Geometry: final body of the model. Coordinates: model frame, mm. A direction names the side the tool comes from. Round coordinates to 2 decimals unless told otherwise and drop trailing zeros. Write each loop counter-clockwise with the first axis right and the second up, starting at its lowest first coordinate (ties: lowest second). Pieces come first, ordered by that corner, then holes. Notation, with made-up numbers: M -33.75,34 L -22.75,34 A19 cw -22.75,47 Z; hole C 61,72 d10. An arc over 180 degrees is marked long. Put each result on its own line as item: value. Start each with the question number.
```python
from build123d import *

# Parameters (mm, degrees)
SKETCH041_W            = 50
SKETCH041_H            = 4.45
PAD014_DEPTH           = 80
PAD013_DEPTH           = 8
SKETCH042_R            = 3
POCKET011_DEPTH        = 5
PAD011_DEPTH           = 6.5
CHAMFER_SIZE           = 2
SKETCH020_W            = 32
SKETCH020_H            = 40
POCKET004_DEPTH        = 4.5
SKETCH021_W            = 16
SKETCH021_H            = 13
POCKET005_DEPTH        = 3
POCKET006_DEPTH        = 2
PAD012_DEPTH           = 2.5
POCKET007_DEPTH        = 5
POCKET008_DEPTH        = 6.501
LINEARPATTERN001_COUNT = 6
LINEARPATTERN001_PITCH = 2.8
POCKET009_DEPTH        = 6.501
POCKET009_DEPTH_BACK   = 6.501
LINEARPATTERN002_COUNT = 6
LINEARPATTERN002_PITCH = 3.2


with BuildPart() as separation_top:
    # Sketch041 → Pad014 (new body)
    with BuildSketch(Plane.XZ.offset(2)):
        with Locations((0, 4.775)):
            Rectangle(SKETCH041_W, SKETCH041_H)
    extrude(amount=-PAD014_DEPTH)

    # AdditivePipe: sweep along a path in Sketch033
    with BuildLine(Plane.XY) as additivepipe_path:
        Line((5.5, 0.7), (15.664513, 0.7))
        ThreePointArc((15.664513, 0.7), (16.796157, 1.050945), (17.530656, 1.980617))
        ThreePointArc((17.530656, 1.980617), (20.610558, 39.551278), (2.853097, 72.80354))
        ThreePointArc((2.853097, 72.80354), (1e-05, 74), (-2.853084, 72.803553))
        ThreePointArc((-2.853084, 72.803553), (-20.610556, 39.551287), (-17.530656, 1.980617))
        ThreePointArc((-17.530656, 1.980617), (-16.796157, 1.050945), (-15.664513, 0.7))
        Line((-15.664513, 0.7), (-5.5, 0.7))
    # Sketch032 → AdditivePipe (sweep)
    with BuildSketch(Plane.YZ):
        Polygon((75.182615, 3), (72.817385, 3), (73.75, 1), (74.25, 1), align=None)
    sweep(path=additivepipe_path.line)

    # Sketch040 → Pad013 (join)
    with BuildSketch(Plane.XY.offset(-2)):
        with BuildLine():
            ThreePointArc((-4.584919, 45.32271), (-5.584919, 44.32271), (-4.584919, 43.32271))
            Line((-4.584919, 43.32271), (4.584919, 43.32271))
            ThreePointArc((4.584919, 43.32271), (5.584919, 44.32271), (4.584919, 45.32271))
            Line((4.584919, 45.32271), (-4.584919, 45.32271))
        make_face()
    extrude(amount=PAD013_DEPTH)

    # Sketch042 → Pocket011 (cut)
    with BuildSketch(Plane.XY):
        with Locations((19, 20)):
            Circle(SKETCH042_R)
        with Locations((-19, 20)):
            Circle(SKETCH042_R)
        with Locations((0, 70)):
            Circle(SKETCH042_R)
    extrude(amount=POCKET011_DEPTH, mode=Mode.SUBTRACT)


with BuildPart() as top_housing:
    # Sketch019 → Pad011 (new body, symmetric)
    with BuildSketch(Plane.XY):
        with BuildLine():
            ThreePointArc((4.279646, 74.20531), (0, 76), (-4.279646, 74.20531))
            ThreePointArc((-4.279646, 74.20531), (-22.568944, 39.95714), (-19.396798, 1.261235))
            ThreePointArc((-19.396798, 1.261235), (-17.9278, -0.59811), (-15.664513, -1.3))
            Line((15.664513, -1.3), (-15.664513, -1.3))
            ThreePointArc((15.664513, -1.3), (17.927792, -0.598116), (19.396791, 1.261217))
            ThreePointArc((19.396791, 1.261217), (22.568946, 39.95713), (4.279646, 74.20531))
        make_face()
    extrude(amount=PAD011_DEPTH, both=True)

    # Chamfer
    chamfer_edges = [top_housing.edges().sort_by_distance(p)[0] for p in [
        (0, -1.3, 6.5),
        (0, -1.3, -6.5),
    ]]
    chamfer(chamfer_edges, length=CHAMFER_SIZE)

    # Sketch020 → Pocket004 (cut)
    with BuildSketch(Plane.XY):
        with Locations((0, 20)):
            Rectangle(SKETCH020_W, SKETCH020_H)
    extrude(amount=POCKET004_DEPTH, mode=Mode.SUBTRACT)

    # Sketch021 → Pocket005 (cut)
    with BuildSketch(Plane.XY):
        with Locations((0, 57)):
            Rectangle(SKETCH021_W, SKETCH021_H)
    extrude(amount=POCKET005_DEPTH, mode=Mode.SUBTRACT)

    # Sketch022 → Pocket006 (cut, symmetric)
    with BuildSketch(Plane.XY):
        with BuildLine():
            ThreePointArc((-6.35, 54.4), (-8.125922, 53.319838), (-7.98356, 51.246101))
            ThreePointArc((-14.445285, 32.796789), (-6.459474, 40.356063), (-7.98356, 51.246101))
            ThreePointArc((-14.445285, 32.796789), (-15.279151, 32.221131), (-15.6, 31.26))
            Line((-15.6, 8.4), (-15.6, 31.26))
            ThreePointArc((-15.6, 8.4), (-15.131371, 7.268629), (-14, 6.8))
            Line((14, 6.8), (-14, 6.8))
            ThreePointArc((14, 6.8), (15.131371, 7.268629), (15.6, 8.4))
            Line((15.6, 31.26), (15.6, 8.4))
            ThreePointArc((15.6, 31.26), (15.279151, 32.221131), (14.445285, 32.796789))
            ThreePointArc((7.98356, 51.246101), (6.459474, 40.356063), (14.445285, 32.796789))
            ThreePointArc((7.98356, 51.246101), (8.125922, 53.319838), (6.35, 54.4))
            Line((6.35, 54.4), (-6.35, 54.4))
        make_face()
    extrude(amount=POCKET006_DEPTH, both=True, mode=Mode.SUBTRACT)

    # Sketch039 → Pad012 (join)
    with BuildSketch(Plane.XY.offset(-0.5)):
        with BuildLine():
            ThreePointArc((-4.584919, 45.32271), (-5.584919, 44.32271), (-4.584919, 43.32271))
            Line((-4.584919, 43.32271), (4.584919, 43.32271))
            ThreePointArc((4.584919, 43.32271), (5.584919, 44.32271), (4.584919, 45.32271))
            Line((4.584919, 45.32271), (-4.584919, 45.32271))
        make_face()
    extrude(amount=PAD012_DEPTH)

    # Sketch023 → Pocket007 (cut, symmetric)
    with BuildSketch(Plane.XZ):
        with BuildLine():
            ThreePointArc((-3, 3.9), (-4.5, 2.4), (-3, 0.9))
            Line((-3, 0.9), (2.5, 0.9))
            ThreePointArc((2.5, 0.9), (4, 2.4), (2.5, 3.9))
            Line((2.5, 3.9), (-3, 3.9))
        make_face()
    extrude(amount=POCKET007_DEPTH, both=True, mode=Mode.SUBTRACT)

    # Sketch025 → Pocket008 (cut, through all)
    with BuildSketch(Plane.XY):
        with BuildLine():
            ThreePointArc((-6.25, 32.5), (-7, 33.25), (-7.75, 32.5))
            Line((-7.75, 32.5), (-7.75, 13.5))
            ThreePointArc((-7.75, 13.5), (-7, 12.75), (-6.25, 13.5))
            Line((-6.25, 13.5), (-6.25, 32.5))
        make_face()
    pocket008 = extrude(amount=POCKET008_DEPTH, mode=Mode.SUBTRACT)

    # LinearPattern001: Pocket008 ×6
    with Locations(*[(i * LINEARPATTERN001_PITCH, 0, 0) for i in range(1, LINEARPATTERN001_COUNT)]):
        add(pocket008, mode=Mode.SUBTRACT)

    # Sketch026 → Pocket009 (cut, two sides)
    with BuildSketch(Plane.XY) as pocket009_sk:
        with BuildLine():
            ThreePointArc((-7, 65), (-8, 66), (-9, 65))
            Line((-9, 65), (-9, 56))
            ThreePointArc((-9, 56), (-8, 55), (-7, 56))
            Line((-7, 56), (-7, 65))
        make_face()
    pocket009 = extrude(amount=-POCKET009_DEPTH, mode=Mode.SUBTRACT) + extrude(pocket009_sk.sketch, amount=POCKET009_DEPTH_BACK, mode=Mode.SUBTRACT)

    # LinearPattern002: Pocket009 ×6
    with Locations(*[(i * LINEARPATTERN002_PITCH, 0, 0) for i in range(1, LINEARPATTERN002_COUNT)]):
        add(pocket009, mode=Mode.SUBTRACT)

    # Sketch027 → Groove (revolve, cut)
    with BuildSketch(Plane.XZ.offset(-20)):
        Polygon((19, 6.7), (19, -5.8), (19.4, -5.8), (20.8, 5.2), (22.3, 6.7), align=None)
    groove = revolve(axis=Axis((19, 20, 6.7), (0, 0, 1)), mode=Mode.SUBTRACT)

    # Mirrored: Groove across YZ
    add(groove.mirror(Plane.YZ), mode=Mode.SUBTRACT)

    # Sketch028 → Groove001 (revolve, cut)
    with BuildSketch(Plane.XZ.offset(-70)):
        Polygon((0, 6.7), (0, -5.8), (0.4, -5.8), (1.8, 5.2), (3.3, 6.7), align=None)
    revolve(axis=Axis((0, 70, 6.7), (0, 0, 1)), mode=Mode.SUBTRACT)

    # Common: intersect Separation top
    add(separation_top.part, mode=Mode.INTERSECT)


solid = top_housing.part
```
1) Ray query, probe 1 along X at (y, z) = (44.5, 1.25); probe 2 along Z at (x, y) = (4.5, 7); probe 3 along X at (y, z) = (70, 2). Return the intervals inside material, ascending.
2) Section B-B, the plane y = 15.5. Give the number of separate pieces and of enclosed holes in the cut face, and give its area (3 significant figures).
3) First-contact query: pin 1 (0.6 mm diameter, centred on y = 21.5, z = 5, fed in from +X); pin 2 (4 mm diameter, centred on x = 0.5, y = 56, fed in from -Z); pin 3 (3 mm diameter, centred on x = 2.5, y = 14.5, fed in from -Z); pin 4 (10 mm diameter, centred on x = 4.5, y = 15, fed in from +Z). Flat tips, straight axial feed; report the tip coordinate or a pass-through.
4) Draft query along X for faces 4 (the face through (-0.2, 0, 4.1)), 5 (the face through (-17.955, -0.579, 3.539)), 6 (the face through (12, 61, 1)), 7 (the face through (1.42, 33.25, 5.49)). Return one class per face: +X half, -X half, draft (parallel to the pull), parting line (faces both ways), or undercut.
5) Section A-A, the plane z = 0.25. Output: boundary loops of the cut face in (x, y), and give its area (3 significant figures).
6) Access query for faces 1 (the face through (-22.455, 40.496, 3.539)), 2 (the face through (-5.8, 61, 5)), 3 (the face through (-0.65, 67.07, 3.76)). Directions: +Z, -Z, +X, -X, +Y, -Y. A direction counts if a zero-diameter tool reaches every point of the face in a straight line with its end or side. Return the directions, or none.
Solved:
1. probe 1: x = -19.77 to -19, -5.57 to 5.57, 19 to 19.77
1. probe 2: z = 4.5 to 6.5
1. probe 3: x = -6.4 to -4.5, 4.5 to 6.4
2. separate pieces: 7
2. enclosed holes: 0
2. area: 103 mm2
3. pin 1: stops at x = 23.65
3. pin 2: stops at z = 3
3. pin 3: stops at z = 4.5
3. pin 4: stops at z = 6.5
4. face 4: undercut
4. face 5: -X half
4. face 6: draft
4. face 7: undercut
5. outline: M -4.58,43.32 L 4.58,43.32 A1 ccw 4.58,45.32 L -4.58,45.32 A1 ccw Z
5. area: 21.5 mm2
6. face 1: +Z, -Z, -X
6. face 2: +Z, -Z
6. face 3: -Z
